Geometry check sheet. Reference: the model listing, model coordinates, mm. A direction names the side the tool comes from. Round coordinates to 2 decimals unless told otherwise and drop trailing zeros. Write each loop counter-clockwise with the first axis right and the second up, starting at its lowest first coordinate (ties: lowest second). Pieces come first, ordered by that corner, then holes.
Item 1: Cross-section at A-A (x = 0). Enter the section's corners in (y, z), then the cut area to 3 significant figures.
Item 2: Scan lines: probe 1 along X at (y, z) = (0, 3.25); probe 2 along X at (y, z) = (-8, 7); probe 3 along X at (y, z) = (5, 8.5). Record each from-to range of solid material in increasing order.
Item 3: Cross-section at B-B (y = 0). Enter the section's corners in (x, z).
Item 4: Draft check along Y on faces 3 (the face through (0.044, 22.385, 4.93)), 4 (the face through (-22.385, 0.044, 4.93)), 5 (the face through (0, 10, 5)). Enter one of: pulls with the +Y half, pulls with the -Y half, needs draft (parallel to the pull), parting line crosses it, or undercut.
Item 5: Depth check by flat-ended pin: P1, Ø13.5, axis at x = 0, y = 0, coming from the +Z side; P2, Ø5, axis at y = 10, z = 3.5, coming from the -X side; P3, Ø0.8, axis at y = 8, z = 5.5, coming from the -X side; P4, Ø1.7, axis at y = 7.5, z = 7, coming from the +X side. Enter the tip coordinate at first touch or a pass-through.
Item 6: Cross-section at C-C (y = -10). Enter the section's corners in (x, z), then the cut area to 3 significant figures.
Item 7: Cross-section at D-D (z = 3.5). Enter the section's corners in (x, y).
Item 8: Access from +Z, -Z, +X, -X, +Y, -Y to the whole of each face (thin tool, end or side, straight path). Record for faces 1 (the face through (-2.5, 8, 5)), 2 (the face through (11.89, -12.15, 4.93)).
from build123d import *

# Parameters (mm, degrees)
EXTRUDE_1_DEPTH    = 10
HOLE_WIZARD_M4_1_D = 4.3


with BuildPart() as part:
    # ｽｹｯﾁ1 → ﾎﾞｽ - 押し出し1 (new body)
    with BuildSketch(Plane.XY):
        with BuildLine():
            Line((-21.213203436, -2.828427125), (-2.828427125, -21.213203436))
            ThreePointArc((-2.828427125, -21.213203436), (0, -22.384776311), (2.828427125, -21.213203436))
            Line((2.828427125, -21.213203436), (21.213203436, -2.828427125))
            ThreePointArc((21.213203436, -2.828427125), (22.384776311, 0), (21.213203436, 2.828427125))
            Line((21.213203436, 2.828427125), (2.828427125, 21.213203436))
            ThreePointArc((2.828427125, 21.213203436), (0, 22.384776311), (-2.828427125, 21.213203436))
            Line((-2.828427125, 21.213203436), (-21.213203436, 2.828427125))
            ThreePointArc((-21.213203436, 2.828427125), (-22.384776311, 0), (-21.213203436, -2.828427125))
        make_face()
        with BuildLine():
            Line((-2.5, 8.585786438), (-2.5, 7.071067812))
            ThreePointArc((-2.5, 7.071067812), (0, -7.5), (2.5, 7.071067812))
            Line((2.5, 7.071067812), (2.5, 8.585786438))
            ThreePointArc((2.5, 8.585786438), (2.5, 10), (1.085786438, 10))
            Line((1.085786438, 10), (-1.085786438, 10))
            ThreePointArc((-1.085786438, 10), (-2.5, 10), (-2.5, 8.585786438))
        make_face(mode=Mode.SUBTRACT)
    extrude(amount=EXTRUDE_1_DEPTH)

    # Hole Wizard M4 _1 (through all)
    with Locations(Plane(origin=(-8.838834765, 8.838834765, 10), x_dir=(1, 0, 0), z_dir=(0, 0, 1))):
        with Locations((0, 0), (17.67766953, 0), (17.67766953, -17.67766953), (0, -17.67766953)):
            Hole(HOLE_WIZARD_M4_1_D / 2)


solid = part.part
Resolved:
1. outline: (-22.38, 0) - (-7.5, 0) - (-7.5, 10) - (-22.38, 10) - close; (10, 0) - (22.38, 0) - (22.38, 10) - (10, 10) - close
1. area: 273 mm2
2. probe 1: x = -22.38 to -7.5, 7.5 to 22.38
2. probe 2: x = -16.04 to -10.82, -6.86 to 6.86, 10.82 to 16.04
2. probe 3: x = -19.04 to -5.59, 5.59 to 19.04
3. outline: (-22.38, 0) - (-7.5, 0) - (-7.5, 10) - (-22.38, 10) - close; (7.5, 0) - (22.38, 0) - (22.38, 10) - (7.5, 10) - close
4. face 3: pulls with the +Y half
4. face 4: parting line crosses it
4. face 5: undercut
5. P1: passes through
5. P2: stops at x = -16.54
5. P3: stops at x = -16.44
5. P4: stops at x = 17.39
6. outline: (-14.04, 0) - (-10.65, 0) - (-10.65, 10) - (-14.04, 10) - close; (-7.03, 0) - (7.03, 0) - (7.03, 10) - (-7.03, 10) - close; (10.65, 0) - (14.04, 0) - (14.04, 10) - (10.65, 10) - close
6. area: 208 mm2
7. outline: (-21.21, -2.83) - (-2.83, -21.21) arc R4 ccw to (2.83, -21.21) - (21.21, -2.83) arc R4 ccw to (21.21, 2.83) - (2.83, 21.21) arc R4 ccw to (-2.83, 21.21) - (-21.21, 2.83) arc R4 ccw to start; hole circle Ø4.3 at (-8.84, -8.84); hole circle Ø4.3 at (-8.84, 8.84); hole (-2.5, 7.07) arc R7.5 ccw (long way) to (2.5, 7.07) - (2.5, 8.59) arc R1 ccw to (1.09, 10) - (-1.09, 10) arc R1 ccw to (-2.5, 8.59) - close; hole circle Ø4.3 at (8.84, -8.84); hole circle Ø4.3 at (8.84, 8.84)
8. face 1: +Z, -Z
8. face 2: +Z, -Z, +X, -Y
